The listing builds one solid part. Answer for the finished solid, in the listing's coordinates (mm). Face numbers are marked on the shaded views. A direction names the side the tool comes from. Coordinates: 2 decimals unless noted, no trailing zeros. Order: outer loops, then holes, each group sorted by start corner. A loop starts at its lowest first (then second) coordinate and runs counter-clockwise, first axis right, second up. Notation, with made-up numbers: M -38.75,85 L -32.75,85 A25 ccw -32.75,99 Z; hole C 65.25,64 d7. An arc over 180 degrees is marked long. One line per item, written item: value. Start each with the question number.
Q1. Straight lines are drawn through the part: line 1 along X through (y, z) = (1.75, 3.25); line 2 along Y through (x, z) = (-16, 0.25); line 3 along Y through (x, z) = (8, -2). For each, find the intervals that lie inside material, in ascending order. Write a range as [from, to].
Q2. Each of these flat-tipped pins is pushed along its axis until it touches: pin 1 Ø2 at (y, z) = (-3.5, 2.5) entering from +X; pin 2 Ø3 at (x, z) = (-15, 1.5) entering from -Y (3 decimals); pin 3 Ø2 at (x, y) = (16.5, -2) entering from -Z; pin 4 Ø1 at (x, y) = (2.5, -4) entering from -Z. Where does it stop, or does it pass through?
Q3. For the marked faces 1 and 2, determine the directions among +Z, -Z, +X, -X, +Y, -Y from which every point of the face is accessible in a straight line to the end or side of a thin tool.
Q4. The part is cut by section A-A on x = 1. Give the vertices of the cut face in (y, z) (3 decimals).
```python
from build123d import *

# Parameters (mm, degrees)
SKETCH5_R           = 3.175
BOSS_EXTRUDE3_DEPTH = 38.1
CHAMFER1_SIZE       = 0.77724
BOSS_EXTRUDE4_DEPTH = 3.96875
SKETCH8_OUTSIDE_W   = 171.38
SKETCH8_OUTSIDE_H   = 173.1
SKETCH8_OUTSIDE_R   = 5.55625
CUT_EXTRUDE3_DEPTH  = 43.06875
CUT_EXTRUDE3_TAPER  = 60
CUT_EXTRUDE4_DEPTH  = 0.254
CIRPATTERN1_COUNT   = 3


with BuildPart() as part:
    # Sketch5 → Boss-Extrude3 (new body)
    with BuildSketch(Plane(origin=(21.034375, 0, 0), x_dir=(0, 0, -1), z_dir=(1, 0, 0))):
        Circle(SKETCH5_R)
    extrude(amount=-BOSS_EXTRUDE3_DEPTH)

    # Chamfer1
    chamfer1_edges = [part.edges().sort_by_distance(p)[0] for p in [
        (21.034375, 0, 3.175),
    ]]
    chamfer(chamfer1_edges, length=CHAMFER1_SIZE)

    # Sketch6 → Boss-Extrude4 (add)
    with BuildSketch(Plane.ZY.offset(17.065625)):
        Polygon((5.55625, 3.207902433), (0, 6.415804866), (-5.55625, 3.207902433), (-5.55625, -3.207902433), (0, -6.415804866), (5.55625, -3.207902433), align=None)
    extrude(amount=BOSS_EXTRUDE4_DEPTH)

    # Sketch8 outside → Cut-Extrude3 (cut, through all)
    with BuildSketch(Plane.ZY.offset(21.034375)):
        Rectangle(SKETCH8_OUTSIDE_W, SKETCH8_OUTSIDE_H)
        Circle(SKETCH8_OUTSIDE_R, mode=Mode.SUBTRACT)
    extrude(amount=-CUT_EXTRUDE3_DEPTH, taper=CUT_EXTRUDE3_TAPER, mode=Mode.SUBTRACT)

    # Sketch12 → Cut-Extrude4 (cut)
    with BuildSketch(Plane.ZY.offset(21.034375)):
        with BuildLine():
            Line((0.1666875, 4.2783125), (0.1666875, 2.3891875))
            ThreePointArc((0.1666875, 2.3891875), (0, 2.2225), (-0.1666875, 2.3891875))
            Line((-0.1666875, 2.3891875), (-0.1666875, 4.2783125))
            ThreePointArc((-0.1666875, 4.2783125), (0, 4.445), (0.1666875, 4.2783125))
        make_face()
    cut_extrude4 = extrude(amount=-CUT_EXTRUDE4_DEPTH, mode=Mode.SUBTRACT)

    # CirPattern1: Cut-Extrude4 ×3 about axis
    cirpattern1_axis = Axis((0, 0, 0), (1, 0, 0))
    for i in range(1, CIRPATTERN1_COUNT):
        add(cut_extrude4.rotate(cirpattern1_axis, i * 360 / CIRPATTERN1_COUNT), mode=Mode.SUBTRACT)


solid = part.part
```
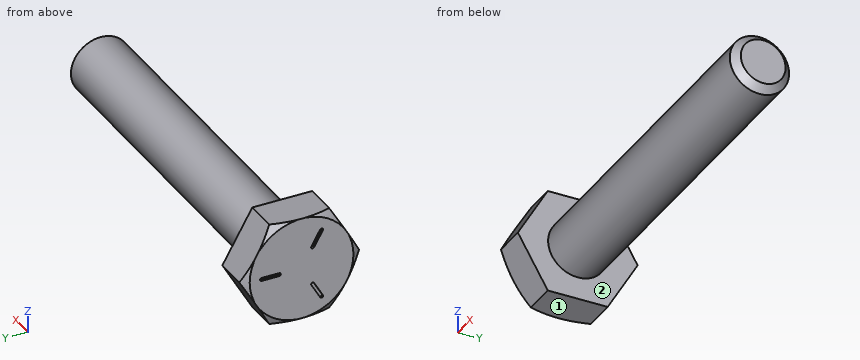
Output:
1. line 1: x = [-21.03, -17.07]
1. line 2: y = [-3.17, 3.17]
1. line 3: y = [-2.47, 2.47]
2. pin 1: stops at x = -17.07
2. pin 2: stops at y = -3.175
2. pin 3: stops at z = -3.01
2. pin 4: passes through
3. face 1: -Z, +X, -X, +Y, -Y
3. face 2: +X
4. outline: C 0,0 d6.35
